For this review, use the dimensioned drawing (mm, ordinates from the lowest corner) and the shaded views. Coordinates: 2 decimals unless noted, no trailing zeros. Order: outer loops, then holes, each group sorted by start corner. A loop starts at its lowest first (then second) coordinate and runs counter-clockwise, first axis right, second up. Notation, with made-up numbers: M -28.75,-4 L 8.25,-4 A24 cw 8.25,31 Z; hole C -27,-32 d2. An arc over 180 degrees is marked long. Answer as CSV lines item,"result". Start each with the question number.
Q1. Consider section A-A on y = 20. Write out the cut boundary in (x, z), and give its area (3 significant figures).
Q2. Consider section C-C on z = 1.05. Write out the cut boundary in (x, y), and give its area (3 significant figures).
Q3. For P1, Ø3.5, axis at x = 10, y = 140, coming from the +Z side, flat-tipped, find the tip position at first contact; note if it passes through.
Q4. Wall thickness on L1, parallel to X at y = 200, z = 1.15; L2, parallel to X at y = 201, z = 3.15: over which ranges is each line inside the solid? List them lowest first. Write a range as [from, to].
Q5. Consider section B-B on x = 10. Write out the cut boundary in (y, z), and give its area (3 significant figures).
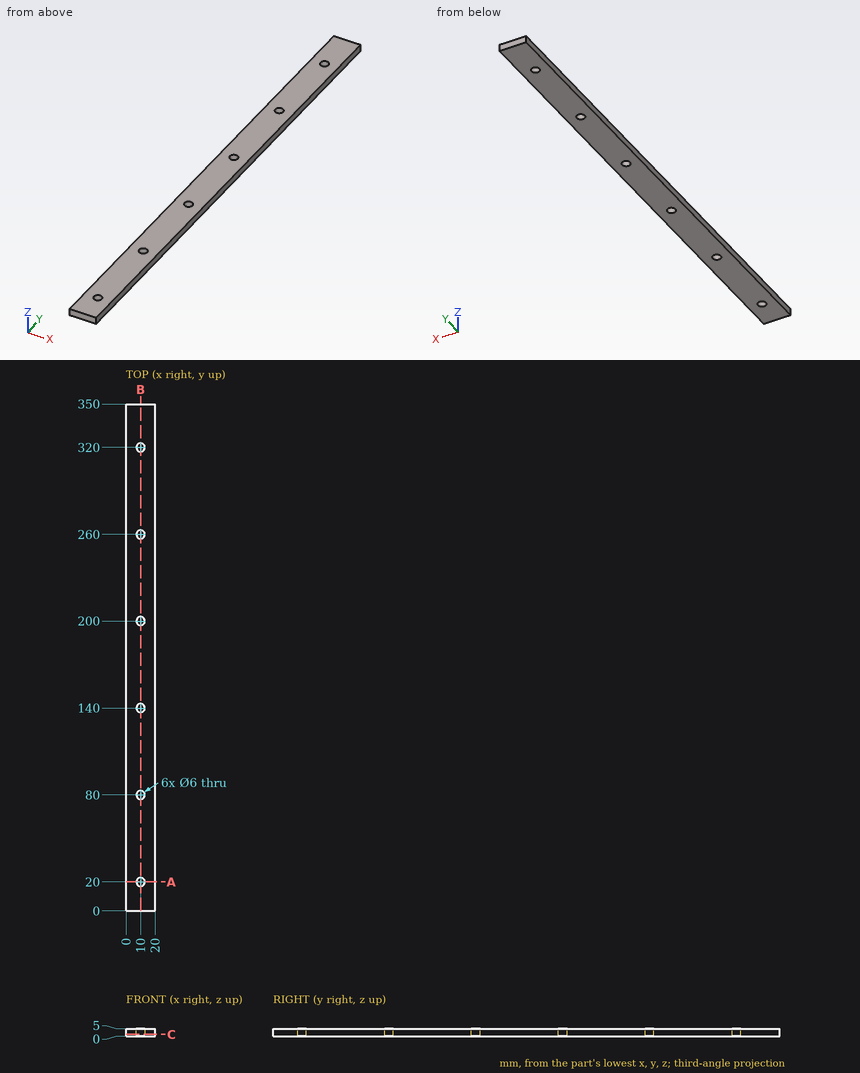
Evaluation:
1,outline,"M 0,0 L 7,0 L 7,5 L 0,5 Z; M 13,0 L 20,0 L 20,5 L 13,5 Z"
1,area,"70.0 mm²"
2,outline,"M 0,0 L 20,0 L 20,350 L 0,350 Z; hole C 10,20 d6; hole C 10,80 d6; hole C 10,140 d6; hole C 10,200 d6; hole C 10,260 d6; hole C 10,320 d6"
2,area,"6,830 mm²"
3,P1,"passes through"
4,L1,"x = [0, 7], [13, 20]"
4,L2,"x = [0, 7.17], [12.83, 20]"
5,outline,"M 0,0 L 17,0 L 17,5 L 0,5 Z; M 23,0 L 77,0 L 77,5 L 23,5 Z; M 83,0 L 137,0 L 137,5 L 83,5 Z; M 143,0 L 197,0 L 197,5 L 143,5 Z; M 203,0 L 257,0 L 257,5 L 203,5 Z; M 263,0 L 317,0 L 317,5 L 263,5 Z; M 323,0 L 350,0 L 350,5 L 323,5 Z"
5,area,"1,570 mm²"
